Geometry: final body of the model. Coordinates: model frame, mm. Give positions to 0.01 mm unless a question says otherwise; leave off trailing zeros. Write each loop counter-clockwise with the first axis right and the second up, starting at its lowest first coordinate (ties: lowest second). Pieces come first, ordered by that corner, then holes. Notation, with made-up numbers: (44.25, 31.25) - (49.25, 31.25) arc R29 cw to (49.25, 55.25) - close; hole circle Ø9 at (31.5, -25.75). An arc over 180 degrees is marked (long way). Use CSV: the item, a comma, the result in double quotes. Start each with the question number.
(1) Section B-B on y = -7.5. Output: boundary loops of the cut face in (x, z).
(2) Line query: probe 1 along Y at (x, z) = (-1.25, -0.1); probe 2 along Y at (x, z) = (3.5, 0.2). Output: solid intervals per line, ascending. Write a range as [from, to].
(3) Section C-C on x = 1.25. Output: boundary loops of the cut face in (y, z).
(4) Section A-A on z = -0.45. Count the separate pieces of the cut face and the enclosed holes in it, and give its area (3 significant figures).
from build123d import *

# Parameters (mm, degrees)
SKETCH1_W           = 18
SKETCH1_H           = 15.5
BOSS_EXTRUDE1_DEPTH = 0.75
SKETCH2_R           = 0.5
CUT_EXTRUDE1_DEPTH  = 1.5


with BuildPart() as part:
    # Sketch1 → Boss-Extrude1 (new, symmetric)
    with BuildSketch(Plane(origin=(0, 0, 0), x_dir=(0, 1, 0), z_dir=(0, 0, 1))):
        Rectangle(SKETCH1_W, SKETCH1_H)
    extrude(amount=BOSS_EXTRUDE1_DEPTH, both=True)

    # Sketch2 → Cut-Extrude1 (cut)
    with BuildSketch(Plane.XY.offset(0.75)):
        with Locations((-6.25, -7.5)):
            Circle(SKETCH2_R)
        with Locations((-3.75, -7.5)):
            Circle(SKETCH2_R)
        with Locations((-1.25, -7.5)):
            Circle(SKETCH2_R)
        with Locations((1.25, -7.5)):
            Circle(SKETCH2_R)
        with Locations((3.75, -7.5)):
            Circle(SKETCH2_R)
        with Locations((6.25, -7.5)):
            Circle(SKETCH2_R)
    cut_extrude1 = extrude(amount=-CUT_EXTRUDE1_DEPTH, mode=Mode.SUBTRACT)

    # Mirror1: Cut-Extrude1 across plane
    add(cut_extrude1.mirror(Plane.ZX), mode=Mode.SUBTRACT)


solid = part.part
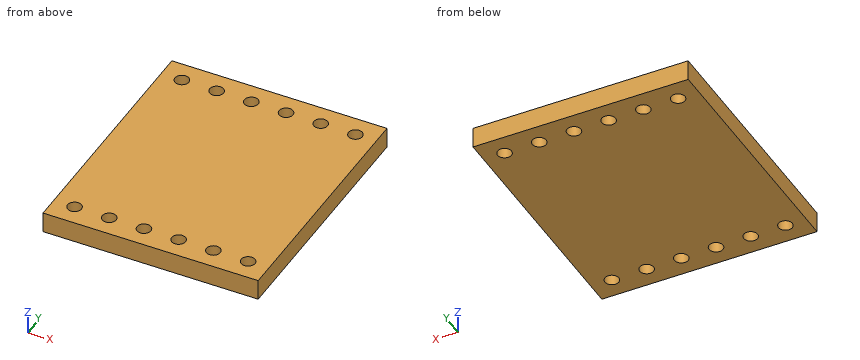
Check values:
1,outline,"(-7.75, -0.75) - (-6.75, -0.75) - (-6.75, 0.75) - (-7.75, 0.75) - close; (-5.75, -0.75) - (-4.25, -0.75) - (-4.25, 0.75) - (-5.75, 0.75) - close; (-3.25, -0.75) - (-1.75, -0.75) - (-1.75, 0.75) - (-3.25, 0.75) - close; (-0.75, -0.75) - (0.75, -0.75) - (0.75, 0.75) - (-0.75, 0.75) - close; (1.75, -0.75) - (3.25, -0.75) - (3.25, 0.75) - (1.75, 0.75) - close; (4.25, -0.75) - (5.75, -0.75) - (5.75, 0.75) - (4.25, 0.75) - close; (6.75, -0.75) - (7.75, -0.75) - (7.75, 0.75) - (6.75, 0.75) - close"
2,probe 1,"y = [-9, -8], [-7, 7], [8, 9]"
2,probe 2,"y = [-9, -7.93], [-7.07, 7.07], [7.93, 9]"
3,outline,"(-9, -0.75) - (-8, -0.75) - (-8, 0.75) - (-9, 0.75) - close; (-7, -0.75) - (7, -0.75) - (7, 0.75) - (-7, 0.75) - close; (8, -0.75) - (9, -0.75) - (9, 0.75) - (8, 0.75) - close"
4,separate pieces,"1"
4,enclosed holes,"12"
4,area,"270 mm²"
